```python
from build123d import *

# Parameters (mm, degrees)
F0_R     = 11.43
F1_DEPTH = 19.05
F2_R     = 7.749073
F3_DEPTH = 19.05


with BuildPart() as f1:
    # F0 (on Top) → F1 (new body)
    with BuildSketch(Plane.XY):
        Circle(F0_R)
    extrude(amount=F1_DEPTH)

    # F2 (on face) → F3 (cut)
    with BuildSketch(Plane(origin=(0, 0, 0), x_dir=(1, 0, 0), z_dir=(0, 0, -1))):
        Circle(F2_R)
    extrude(amount=-F3_DEPTH, mode=Mode.SUBTRACT)

    # F4 (on Front) → F5 (revolve)
    with BuildSketch(Plane.XZ):
        Polygon((0, -22.978624), (11.502104, 0), (0, 0), align=None)
    revolve(axis=Axis((0, 0, -11.489312), (0, 0, 1)))

    # F6 (on Right) → F7 (revolve, cut)
    with BuildSketch(Plane.YZ):
        Polygon((0, 0), (-8.085498, 0), (0, -27.366927), align=None)
    revolve(axis=Axis((0, 0, -13.683463), (0, 0, 1)), mode=Mode.SUBTRACT)


solid = f1.part
```
Work out the finished part from the listing and answer in its coordinate system (mm). Round coordinates to 2 decimals unless told otherwise and drop trailing zeros. Order: outer loops, then holes, each group sorted by start corner. A loop starts at its lowest first (then second) coordinate and runs counter-clockwise, first axis right, second up.
Q1. Find the intervals of material crossed by line 1 along Y through (x, z) = (0, 7.75); line 2 along Y through (x, z) = (-6.75, 3); line 3 along X through (y, z) = (7, 1), in increasing order.
Solution:
line 1: y = -11.43 to -7.75, 7.75 to 11.43
line 2: y = -9.22 to -3.81, 3.81 to 9.22
line 3: x = -9.04 to -3.32, 3.32 to 9.04
Q2. A cutting plane is placed at A-A, the plane x = 0. Determine the outline of the cut face in (y, z), then the cut area to 3 significant figures.
Solution:
outline: (-11.5, 0) - (-3.16, -16.66) - (-8.09, 0) - (-7.75, 0) - (-7.75, 19.05) - (-11.43, 19.05) - (-11.43, 0) - close; (3.16, -16.66) - (11.5, 0) - (11.43, 0) - (11.43, 19.05) - (7.75, 19.05) - (7.75, 0) - (8.09, 0) - close
area: 197 mm2
Q3. A cutting plane is placed at C-C, the plane z = 17.5. Determine the outline of the cut face in (x, y), then the cut area to 3 significant figures.
Solution:
outline: circle Ø22.86 at (0, 0); hole circle Ø15.5 at (0, 0)
area: 222 mm2
Q4. Given pin 1 Ø2 at (x, z) = (-3, -9) entering from +Y; pin 2 Ø12 at (y, z) = (6, 15.5) entering from +X; pin 3 Ø12 at (y, z) = (0, -9.5) entering from -X, each flat-ended and moving along its own axis, determine where each tip first touches the part or whether it passes through.
Solution:
pin 1: stops at y = 7
pin 2: stops at x = 11.43
pin 3: stops at x = -9.75
Q5. The mould has two halves that part along X. Classify faces 1 (the conical face through (5.283, 1.664, -11.914)), 2 (the cylindrical face through (-7.74, -0.34, 9.39)), 3 (the flat face through (-2.7, -7.5, 19.05)): pulls with the +X half, pulls with the -X half, needs draft (parallel to the pull), parting line crosses it, or undercut.
Solution:
face 1: parting line crosses it
face 2: undercut
face 3: needs draft
Q6. A cutting plane is placed at D-D, the plane z = -13. Determine the outline of the cut face in (x, y).
Solution:
outline: circle Ø9.99 at (0, 0); hole circle Ø8.49 at (0, 0)
